Read the model definition and answer for the solid it produces. Units are mm, in the model's axes. Face numbers are marked on the shaded views. A direction names the side the tool comes from. Give positions to 0.01 mm unless a question says otherwise; leave off trailing zeros. Write each loop counter-clockwise with the first axis right and the second up, starting at its lowest first coordinate (ties: lowest second). Pieces come first, ordered by that corner, then holes. Notation, with made-up numbers: (62, -22) -> (119, -22) arc R11 cw to (119, -11) -> close; hole circle Ø2 at (-16, -19). An arc over 180 degrees is marked (long way). Answer as CSV lines item,"result". Start each with the question number.
1. Given pin 1 (4 mm diameter, centred on x = -2, y = -2.5, fed in from -Z); pin 2 (1.5 mm diameter, centred on x = -2, z = -1, fed in from +Y), each flat-ended and moving along its own axis, determine where each tip first touches the part or whether it passes through.
2. The part is cut by section B-B, the plane y = 0. Determine the outline of the cut face in (x, z) (3 decimals).
3. The part is cut by section A-A, the plane z = 0. Determine the outline of the cut face in (x, y) (3 decimals), and give its area (3 significant figures).
4. A tool of negligible diameter and unlimited length cuts with its end or side. For the marked faces 5 and 6, from which of +Z, -Z, +X, -X, +Y, -Y can it reach the whole face along a straight path? Write none if from no direction.
5. The part is cut by section D-D, the plane y = -2.5. Determine the outline of the cut face in (x, z), and give its area (3 significant figures).
6. For a pull along X with two mould halves and no side action, classify the marked faces 1, 2, 3 and 4 as pulls with the +X half, pulls with the -X half, needs draft (parallel to the pull), parting line crosses it, or undercut.
7. Find the intervals of material crossed by line 1 (X direction, y = 0, z = -1.5) (3 decimals); line 2 (X direction, y = 0, z = 1.5) (3 decimals); line 3 (X direction, y = -3.5, z = -2), in increasing order.
8. The part is cut by section C-C, the plane x = -10.5. Determine the outline of the cut face in (y, z).
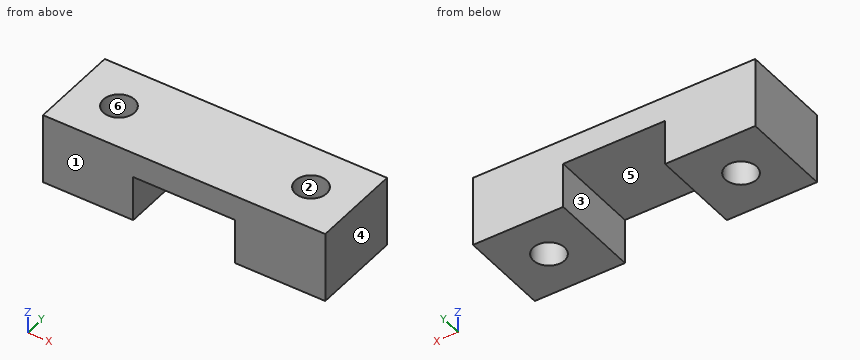
from build123d import *

# Parameters (mm, degrees)
F1_DEPTH = 4.5
F2_R     = 1.55
F3_DEPTH = 7


with BuildPart() as f1:
    # F0 (on Front) → F1 (new body, symmetric)
    with BuildSketch(Plane.XZ):
        Polygon((14, 3.5), (0, 3.5), (-14, 3.5), (-14, -3.5), (-5.05, -3.5), (-5.05, 1), (0, 1), (5.05, 1), (5.05, -3.5), (14, -3.5), align=None)
    extrude(amount=F1_DEPTH, both=True)

    # F2 (on face) → F3 (cut, through all)
    with BuildSketch(Plane(origin=(0, 0, -3.5), x_dir=(1, 0, 0), z_dir=(0, 0, -1))):
        with Locations((9.525, 0)):
            Circle(F2_R)
        with Locations((-9.525, 0)):
            Circle(F2_R)
    extrude(amount=-F3_DEPTH, mode=Mode.SUBTRACT)


solid = f1.part
Results found:
1,pin 1,"stops at z = 1"
1,pin 2,"passes through"
2,outline,"(-14, -3.5) -> (-11.075, -3.5) -> (-11.075, 3.5) -> (-14, 3.5) -> close; (-7.975, -3.5) -> (-5.05, -3.5) -> (-5.05, 1) -> (5.05, 1) -> (5.05, -3.5) -> (7.975, -3.5) -> (7.975, 3.5) -> (-7.975, 3.5) -> close; (11.075, -3.5) -> (14, -3.5) -> (14, 3.5) -> (11.075, 3.5) -> close"
3,outline,"(-14, -4.5) -> (-5.05, -4.5) -> (-5.05, 4.5) -> (-14, 4.5) -> close; (5.05, -4.5) -> (14, -4.5) -> (14, 4.5) -> (5.05, 4.5) -> close; hole circle Ø3.1 at (-9.525, 0); hole circle Ø3.1 at (9.525, 0)"
3,area,"146 mm²"
4,face 5,"-Z, +Y, -Y"
4,face 6,"+Z, -Z"
5,outline,"(-14, -3.5) -> (-5.05, -3.5) -> (-5.05, 1) -> (5.05, 1) -> (5.05, -3.5) -> (14, -3.5) -> (14, 3.5) -> (-14, 3.5) -> close"
5,area,"151 mm²"
6,face 1,"needs draft"
6,face 2,"undercut"
6,face 3,"undercut"
6,face 4,"pulls with the +X half"
7,line 1,"x = -14 to -11.075, -7.975 to -5.05, 5.05 to 7.975, 11.075 to 14"
7,line 2,"x = -14 to -11.075, -7.975 to 7.975, 11.075 to 14"
7,line 3,"x = -14 to -5.05, 5.05 to 14"
8,outline,"(-4.5, -3.5) -> (-1.2, -3.5) -> (-1.2, 3.5) -> (-4.5, 3.5) -> close; (1.2, -3.5) -> (4.5, -3.5) -> (4.5, 3.5) -> (1.2, 3.5) -> close"
